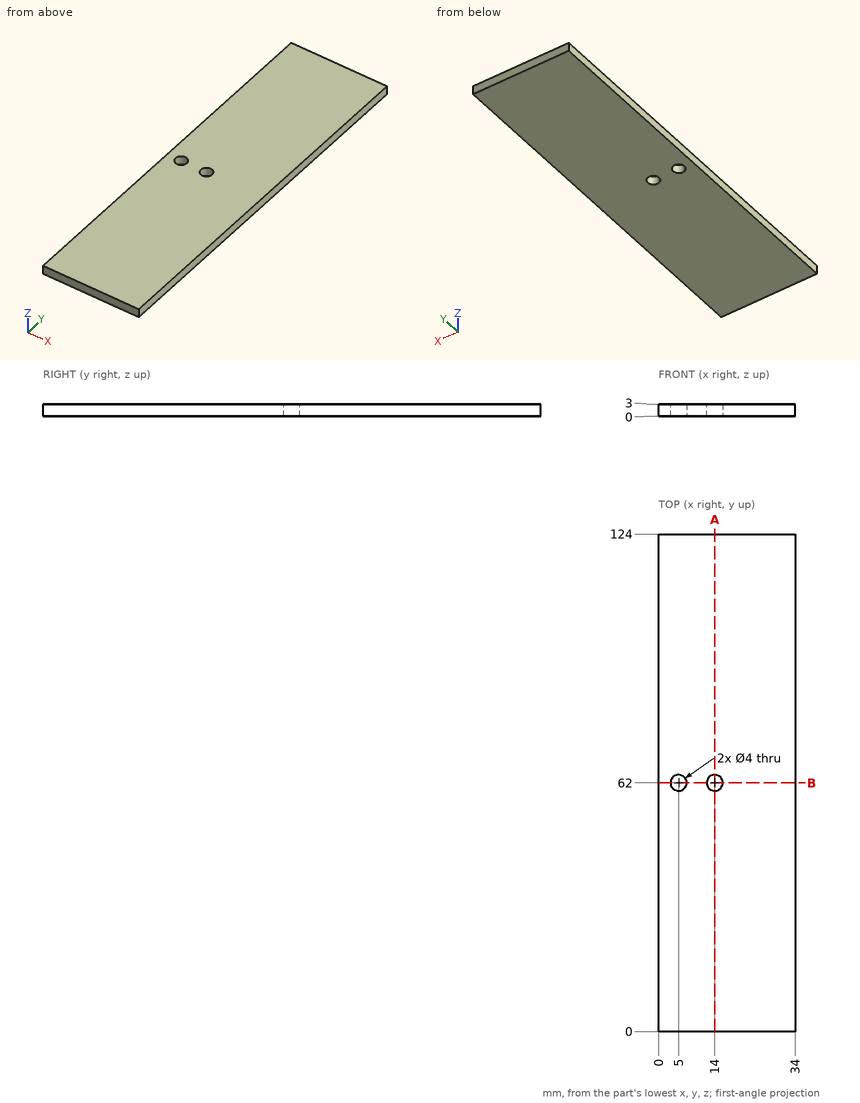
Here's the drawing with two shaded views (mm, measured from the low corner). I have some questions. Coordinates: 2 decimals unless noted, no trailing zeros. Loops run counter-clockwise (first coordinate to the right, second up) from the corner with the lowest first, then second, coordinate; pieces in that order, holes last. Notation, with made-up numbers: (-28.75, 76) -> (-23.75, 76) arc R26 ccw to (-23.75, 97) -> close; hole circle Ø10 at (83, -22). An arc over 180 degrees is marked (long way). Answer in a Markdown table with one row per item.
(1) If I drill on probe 1 along Y at (x, z) = (14, 1.1); probe 2 along Y at (x, z) = (13, 0.85), over which ranges is the centre line in solid material (lowest first)?
Results found:
| item | result |
|---|---|
| probe 1 | y = 0 to 60, 64 to 124 |
| probe 2 | y = 0 to 60.27, 63.73 to 124 |
(2) Imagine slicing it at B-B (y = 62). List the corners of the cut face in (x, z) for me, plus the area to 3 significant figures.
Results found:
| item | result |
|---|---|
| outline | (0, 0) -> (3, 0) -> (3, 3) -> (0, 3) -> close; (7, 0) -> (12, 0) -> (12, 3) -> (7, 3) -> close; (16, 0) -> (34, 0) -> (34, 3) -> (16, 3) -> close |
| area | 78.0 mm^2 |
(3) Imagine slicing it at A-A (x = 14). List the corners of the cut face in (y, z) for me, plus the area to 3 significant figures.
Results found:
| item | result |
|---|---|
| outline | (0, 0) -> (60, 0) -> (60, 3) -> (0, 3) -> close; (64, 0) -> (124, 0) -> (124, 3) -> (64, 3) -> close |
| area | 360 mm^2 |
